Could you check a few things on this model? Use its own coordinates, in mm. A direction names the side the tool comes from. Round coordinates to 2 decimals unless told otherwise and drop trailing zeros. Write each loop counter-clockwise with the first axis right and the second up, starting at its lowest first coordinate (ties: lowest second). Pieces come first, ordered by that corner, then holes. Notation, with made-up numbers: (26.25, 59.5) - (70.25, 59.5) arc R28 ccw to (70.25, 86.5) - close; hole circle Ø5 at (5, 6.25). An arc over 180 degrees is marked (long way). Put each result on its own line as item: value.
from build123d import *

# Parameters (mm, degrees)
SKETCH1_W           = 25.4
SKETCH1_H           = 89.50000007
SKETCH1_R           = 1.75
BOSS_EXTRUDE1_DEPTH = 10.35
SKETCH2_R           = 12.7
SKETCH2_R_2         = 10.5
BOSS_EXTRUDE2_DEPTH = 12.7
SKETCH5_W           = 2
SKETCH5_H           = 8.007473722
CUT_EXTRUDE1_DEPTH  = 12.7
SKETCH6_R           = 6
CUT_EXTRUDE2_DEPTH  = 3
SKETCH7_R           = 2
CUT_EXTRUDE3_DEPTH  = 7.35
SKETCH8_W           = 21.78000007
SKETCH8_H           = 3
CUT_EXTRUDE4_DEPTH  = 2


with BuildPart() as part:
    # Sketch1 → Boss-Extrude1 (new body)
    with BuildSketch(Plane(origin=(0, 0, 0), x_dir=(1, 0, 0), z_dir=(0, 1, 0))):
        with Locations((12.7, 44.750000035)):
            Rectangle(SKETCH1_W, SKETCH1_H)
        with Locations((5, 84.50000007)):
            Circle(SKETCH1_R, mode=Mode.SUBTRACT)
        with Locations((20.4, 84.50000007)):
            Circle(SKETCH1_R, mode=Mode.SUBTRACT)
        with Locations((5, 5)):
            Circle(SKETCH1_R, mode=Mode.SUBTRACT)
        with Locations((20.4, 5)):
            Circle(SKETCH1_R, mode=Mode.SUBTRACT)
    extrude(amount=BOSS_EXTRUDE1_DEPTH)

    # Sketch2 → Boss-Extrude2 (add)
    with BuildSketch(Plane(origin=(0, 10.35, 0), x_dir=(1, 0, 0), z_dir=(0, 1, 0))):
        with Locations((12.7, 47.75000007)):
            Circle(SKETCH2_R)
        with Locations((12.7, 47.75000007)):
            Circle(SKETCH2_R_2, mode=Mode.SUBTRACT)
    extrude(amount=BOSS_EXTRUDE2_DEPTH)

    # Sketch5 → Cut-Extrude1 (cut)
    with BuildSketch(Plane(origin=(0, 23.05, 0), x_dir=(1, 0, 0), z_dir=(0, 1, 0))):
        with Locations((12.7, 58.700520661)):
            Rectangle(SKETCH5_W, SKETCH5_H)
    extrude(amount=-CUT_EXTRUDE1_DEPTH, mode=Mode.SUBTRACT)

    # Sketch6 → Cut-Extrude2 (cut)
    with BuildSketch(Plane(origin=(0, 10.35, 0), x_dir=(1, 0, 0), z_dir=(0, 1, 0))):
        with Locations((12.7, 47.75000007)):
            Circle(SKETCH6_R)
    extrude(amount=-CUT_EXTRUDE2_DEPTH, mode=Mode.SUBTRACT)

    # Sketch7 → Cut-Extrude3 (cut)
    with BuildSketch(Plane(origin=(0, 7.35, 0), x_dir=(1, 0, 0), z_dir=(0, 1, 0))):
        with Locations((12.7, 47.75000007)):
            Circle(SKETCH7_R)
    extrude(amount=-CUT_EXTRUDE3_DEPTH, mode=Mode.SUBTRACT)

    # Sketch8 → Cut-Extrude4 (cut)
    with BuildSketch(Plane(origin=(25.4, 0, 0), x_dir=(0, 0, -1), z_dir=(1, 0, 0))):
        with Locations((47.750000035, 1.5)):
            Rectangle(SKETCH8_W, SKETCH8_H)
    cut_extrude4 = extrude(amount=-CUT_EXTRUDE4_DEPTH, mode=Mode.SUBTRACT)

    # Mirror1: Cut-Extrude4 across plane
    add(cut_extrude4.mirror(Plane.ZY.offset(-12.7)), mode=Mode.SUBTRACT)


solid = part.part
(1) Imagine slicing it at D-D, the plane z = -52.5. List the corners of the cut face in (x, y) for me.
Values found:
outline: (0, 3) - (2, 3) - (2, 0) - (23.4, 0) - (23.4, 3) - (25.4, 3) - (25.4, 10.35) - (24.48, 10.35) - (24.48, 23.05) - (22.06, 23.05) - (22.06, 10.35) - (16.37, 10.35) - (16.37, 7.35) - (9.03, 7.35) - (9.03, 10.35) - (3.34, 10.35) - (3.34, 23.05) - (0.92, 23.05) - (0.92, 10.35) - (0, 10.35) - close
(2) Imagine slicing it at B-B, the plane z = -5. List the corners of the cut face in (x, y) for me.
Values found:
outline: (0, 0) - (3.25, 0) - (3.25, 10.35) - (0, 10.35) - close; (6.75, 0) - (18.65, 0) - (18.65, 10.35) - (6.75, 10.35) - close; (22.15, 0) - (25.4, 0) - (25.4, 10.35) - (22.15, 10.35) - close
(3) Imagine slicing it at C-C, the plane x = 21.25. List the corners of the cut face in (y, z) for me, then the cut area to 3 significant figures.
Values found:
outline: (0, -89.5) - (10.35, -89.5) - (10.35, -86.03) - (0, -86.03) - close; (0, -82.97) - (10.35, -82.97) - (10.35, -57.14) - (23.05, -57.14) - (23.05, -53.84) - (10.35, -53.84) - (10.35, -41.66) - (23.05, -41.66) - (23.05, -38.36) - (10.35, -38.36) - (10.35, -6.53) - (0, -6.53) - close; (0, -3.47) - (10.35, -3.47) - (10.35, 0) - (0, 0) - close
area: 947 mm^2
(4) If we mould it in two halves opening along Z, with no side actions, what happens to faces 1 (the face through (1, 3, -48)), 2 (the face through (4.62, 5.1, -82.79)), 3 (the face through (13.7, 17, -59)), 4 (the face through (13, 5, 0))? For each: pulls with the +Z half, pulls with the -Z half, needs draft (parallel to the pull), parting line crosses it, or undercut.
Values found:
face 1: undercut
face 2: undercut
face 3: needs draft
face 4: pulls with the +Z half
(5) Imagine slicing it at A-A, the plane x = 12.7. List the corners of the cut face in (y, z) for me, then the cut area to 3 significant figures.
Values found:
outline: (0, -89.5) - (10.35, -89.5) - (10.35, -53.75) - (7.35, -53.75) - (7.35, -49.75) - (0, -49.75) - close; (0, -45.75) - (7.35, -45.75) - (7.35, -41.75) - (10.35, -41.75) - (10.35, -37.25) - (23.05, -37.25) - (23.05, -35.05) - (10.35, -35.05) - (10.35, 0) - (0, 0) - close
area: 889 mm^2
(6) For faces 5 (the face through (12.16, 16.61, -35.06)), 6 (the face through (1, 1, -36.86)), 7 (the face through (0, 5, -44)), 8 (the face through (24, 3, -48)), which set-ups out of +Z, -Z, +X, -X, +Y, -Y let a thin tool reach every point of the face, with its end or its side?
Values found:
face 5: +Y
face 6: -X, -Y
face 7: +Z, -Z, -X, +Y, -Y
face 8: +X, -Y
(7) Please list where these lines run through material, in increasing order: probe 1 along X at (y, z) = (5.75, -84.5); probe 2 along Z at (x, y) = (5, 3); probe 3 along X at (y, z) = (18.5, -47.75). Write a range as from..to.
Values found:
probe 1: x = 0..3.25, 6.75..18.65, 22.15..25.4
probe 2: z = -89.5..-86.25, -82.75..-6.75, -3.25..0
probe 3: x = 0..2.2, 23.2..25.4
(8) I'm going to push flat-ended pins straight in: pin 1 (1.8 mm diameter, centred on y = 15, z = -59.5, fed in from -X); pin 2 (9.5 mm diameter, centred on x = 12.7, z = -47.75, fed in from +Y); pin 3 (2.5 mm diameter, centred on y = 1, z = -49, fed in from +X). Where does each tip first touch, or does it pass through?
Values found:
pin 1: stops at x = 6.1
pin 2: stops at y = 7.35
pin 3: stops at x = 23.4
